from build123d import *

# Parameters (mm, degrees)
ESQUISSE1_W                  = 140
ESQUISSE1_H                  = 140
BOSS_EXTRU_1_DEPTH           = 13.5
ENL_V_MAT_EXTRU_3_DEPTH      = 8.5
ENL_V_MAT_EXTRU_1_DEPTH      = 100
R_P_TITION_CIRCULAIRE1_COUNT = 2
R_P_TITION_CIRCULAIRE1_ANGLE = 90
CONG_1_R                     = 10
ESQUISSE3_R                  = 1.5
ENL_V_MAT_EXTRU_2_DEPTH      = 13.5
ESQUISSE5_R                  = 1.5
ENL_V_MAT_EXTRU_4_DEPTH      = 10
ENL_V_MAT_EXTRU_4_DEPTH_BACK = 12.5


with BuildPart() as part:
    # Esquisse1 → Boss.-Extru.1 (new body)
    with BuildSketch(Plane.XY):
        Rectangle(ESQUISSE1_W, ESQUISSE1_H)
        Polygon((65, 12.5), (55, 2.5), (55, 32.5), (65, 42.5), align=None, mode=Mode.SUBTRACT)
        Polygon((65, -12.5), (55, -2.5), (55, -32.5), (65, -42.5), align=None, mode=Mode.SUBTRACT)
        Polygon((12.5, -65), (2.5, -55), (32.5, -55), (42.5, -65), align=None, mode=Mode.SUBTRACT)
        Polygon((-12.5, -65), (-2.5, -55), (-32.5, -55), (-42.5, -65), align=None, mode=Mode.SUBTRACT)
        Polygon((-65, -12.5), (-55, -2.5), (-55, -32.5), (-65, -42.5), align=None, mode=Mode.SUBTRACT)
        Polygon((-65, 12.5), (-55, 2.5), (-55, 32.5), (-65, 42.5), align=None, mode=Mode.SUBTRACT)
        Polygon((-12.5, 65), (-2.5, 55), (-32.5, 55), (-42.5, 65), align=None, mode=Mode.SUBTRACT)
        Polygon((12.5, 65), (2.5, 55), (32.5, 55), (42.5, 65), align=None, mode=Mode.SUBTRACT)
    extrude(amount=BOSS_EXTRU_1_DEPTH)

    # Esquisse4 → Enl_v. mat.-Extru.3 (cut)
    with BuildSketch(Plane.XY.offset(13.5)):
        Polygon((-21.715728753, 50), (-50, 21.715728753), (-50, -21.715728753), (-21.715728753, -50), (21.715728753, -50), (50, -21.715728753), (50, 21.715728753), (21.715728753, 50), align=None)
    extrude(amount=-ENL_V_MAT_EXTRU_3_DEPTH, mode=Mode.SUBTRACT)

    # Esquisse2 → Enl_v. mat.-Extru.1 (cut, symmetric)
    with BuildSketch(Plane(origin=(0, 0, 0), x_dir=(-0.707106781, -0.707106781, 0), z_dir=(-0.707106781, 0.707106781, 0))):
        with BuildLine():
            Line((-6, 14), (6, 14))
            ThreePointArc((6, 14), (0, 8), (-6, 14))
        make_face()
    enl_v_mat_extru_1 = extrude(amount=ENL_V_MAT_EXTRU_1_DEPTH, both=True, mode=Mode.SUBTRACT)

    # R_p_tition circulaire1: Enl_v. mat.-Extru.1 ×2 about axis
    r_p_tition_circulaire1_axis = Axis((0, 0, -62.841973852), (0, 0, 1))
    for i in range(1, R_P_TITION_CIRCULAIRE1_COUNT):
        add(enl_v_mat_extru_1.rotate(r_p_tition_circulaire1_axis, i * R_P_TITION_CIRCULAIRE1_ANGLE / (R_P_TITION_CIRCULAIRE1_COUNT - 1)), mode=Mode.SUBTRACT)

    # Cong_1
    cong_1_edges = [part.edges().sort_by_distance(p)[0] for p in [
        (-70, 70, 4),
        (-70, -70, 4),
        (70, 70, 4),
        (70, -70, 4),
        (-21.715728753, -50, 9.25),
        (21.715728753, -50, 9.25),
        (50, -21.715728753, 9.25),
        (50, 21.715728753, 9.25),
        (21.715728753, 50, 9.25),
        (-21.715728753, 50, 9.25),
        (-50, -21.715728753, 9.25),
        (-50, 21.715728753, 9.25),
    ]]
    fillet(cong_1_edges, radius=CONG_1_R)

    # Esquisse3 → Enl_v. mat.-Extru.2 (cut)
    with BuildSketch(Plane.XY.offset(13.5)):
        with Locations((-60, -44.443650814)):
            Circle(ESQUISSE3_R)
        with Locations((-44.443650814, -60)):
            Circle(ESQUISSE3_R)
        with Locations((-44.443650814, 60)):
            Circle(ESQUISSE3_R)
        with Locations((-60, 44.443650814)):
            Circle(ESQUISSE3_R)
        with Locations((60, 44.443650814)):
            Circle(ESQUISSE3_R)
        with Locations((44.443650814, 60)):
            Circle(ESQUISSE3_R)
        with Locations((44.443650814, -60)):
            Circle(ESQUISSE3_R)
        with Locations((60, -44.443650814)):
            Circle(ESQUISSE3_R)
    extrude(amount=-ENL_V_MAT_EXTRU_2_DEPTH, mode=Mode.SUBTRACT)

    # Esquisse5 → Enl_v. mat.-Extru.4 (cut, two sides)
    with BuildSketch(Plane.XY.offset(5)) as enl_v_mat_extru_4_sk:
        with Locations((-52, 22.5)):
            Circle(ESQUISSE5_R)
        with Locations((-7.000000025, 22.498488866)):
            Circle(ESQUISSE5_R)
        with Locations((-52.000000025, -22.5)):
            Circle(ESQUISSE5_R)
        with Locations((-7.000000025, -22.501511134)):
            Circle(ESQUISSE5_R)
        with Locations((-12.5, 12.5)):
            Circle(ESQUISSE5_R)
        with Locations((12.5, 12.5)):
            Circle(ESQUISSE5_R)
        with Locations((12.5, -12.5)):
            Circle(ESQUISSE5_R)
        with Locations((-12.5, -12.5)):
            Circle(ESQUISSE5_R)
        with Locations((33.837049096, 49.393398282)):
            Circle(ESQUISSE5_R)
        with Locations((49.393398282, 33.837049096)):
            Circle(ESQUISSE5_R)
        with Locations((49.393398282, -33.837049096)):
            Circle(ESQUISSE5_R)
        with Locations((33.837049096, -49.393398282)):
            Circle(ESQUISSE5_R)
        with Locations((-33.837049096, -49.393398282)):
            Circle(ESQUISSE5_R)
        with Locations((-49.393398282, -33.837049096)):
            Circle(ESQUISSE5_R)
        with Locations((-49.393398282, 33.837049096)):
            Circle(ESQUISSE5_R)
        with Locations((-33.837049096, 49.393398282)):
            Circle(ESQUISSE5_R)
    extrude(amount=ENL_V_MAT_EXTRU_4_DEPTH, mode=Mode.SUBTRACT)
    extrude(enl_v_mat_extru_4_sk.sketch, amount=-ENL_V_MAT_EXTRU_4_DEPTH_BACK, mode=Mode.SUBTRACT)


solid = part.part
For this review, take the finished solid that the model builds, in its own axes (mm). A direction names the side the tool comes from. Give positions to 0.01 mm unless a question says otherwise; leave off trailing zeros. Order: outer loops, then holes, each group sorted by start corner. A loop starts at its lowest first (then second) coordinate and runs counter-clockwise, first axis right, second up. Notation, with made-up numbers: (-19.75, 66.5) - (-1.75, 66.5) arc R18 cw to (-1.75, 90.5) - close; hole circle Ø6 at (54.25, 2.25). An arc over 180 degrees is marked (long way). Answer as a JSON object with one key per item and string values. Group by question number.
Item 1: Machinability: for faces 1 (the flat face through (35.701, -36.015, 7.421)), 2 (the flat face through (28, 65, 7)), 3 (the flat face through (-1, 1, 0)), which of the approach directions +Z, -Z, +X, -X, +Y, -Y give a long, thin tool a straight path to every point of the face, cutting with its end or side? Answer none if there is none.
Item 2: Take a section at A-A on x = 29.5. Give the boundary of the cut face in (y, z), and give its area (3 significant figures).
Item 3: Take a section at B-B on z = 3.25. Give the number of separate pieces and of enclosed holes in the cut face, and give its area (3 significant figures).
Item 4: Draft analysis for pull direction X (two halves, no side actions). For faces 4 (the flat face through (58, 1, 13.5)), 5 (the cylindrical face through (66.99, -67.15, 5.34)), 6 (the cylindrical face through (51, -51, 8)), 7 (the flat face through (-70, -1, 7)), state which applies: pulls with the +X half, pulls with the -X half, needs draft (parallel to the pull), parting line crosses it, or undercut.
Item 5: Clearance check with flat-ended pins moving along their axes: pin 1 Ø4 at (x, y) = (49.39, -33.84) entering from -Z; pin 2 Ø4 at (x, y) = (-21.5, -14.5) entering from +Z. State where each tip first meets the part, or that it passes through.
Item 6: Wall thickness on line 1 along Y through (x, z) = (-28.5, 3.25); line 2 along X through (y, z) = (36, 2.75); line 3 along X through (y, z) = (-14, 10.25): over which ranges is each line inside the solid? List them lowest first.
Reported:
{
 "1": {"face 1": "+Z", "face 2": "+Z, -Z", "face 3": "-Z, +X, -X, +Y, -Y"},
 "2": {"outline": "(-70, 0) - (-65, 0) - (-65, 13.5) - (-70, 13.5) - close; (-55, 0) - (55, 0) - (55, 13.5) - (42.22, 13.5) - (42.22, 5) - (-42.22, 5) - (-42.22, 13.5) - (-55, 13.5) - close; (65, 0) - (70, 0) - (70, 13.5) - (65, 13.5) - close", "area": "902 mm^2"},
 "3": {"separate pieces": "1", "enclosed holes": "32", "area": "16,900 mm^2"},
 "4": {"face 4": "needs draft", "face 5": "pulls with the +X half", "face 6": "undercut", "face 7": "pulls with the -X half"},
 "5": {"pin 1": "z = 0", "pin 2": "z = 5"},
 "6": {"line 1": "-70 to -65, -55 to 55, 65 to 70", "line 2": "-70 to -65, -58.5 to 58.5, 65 to 70", "line 3": "-70 to -65, -55 to -50, 50 to 55, 65 to 70"}
}
